Could you check a few things on this model? Use its own coordinates, in mm. A direction names the side the tool comes from. Give positions to 0.01 mm unless a question says otherwise; leave off trailing zeros. Loops run counter-clockwise (first coordinate to the right, second up) from the corner with the lowest first, then second, coordinate; pieces in that order, holes last. Notation, with made-up numbers: (34.5, 43) -> (59.5, 43) arc R30 ccw to (59.5, 71) -> close; hole circle Ø6 at (-24, 33.25). An arc over 180 degrees is marked (long way). Write each question's results on one line, items separated by ' | '. Start each with the question number.
Q1. We'd pull the mould along Y, two halves only. Please class faces 3 (the face through (-1, 1, 0)), 4 (the face through (-2.92, 7.56, 6.65)), 5 (the face through (-16.01, -72.08, 3.45)): released by +Y, released by -Y, zero draft, split by the parting line, or undercut.
Q2. If I drill on line 1 along Y through (x, z) = (0, 6.8); line 2 along Z through (x, y) = (-40.5, 53.5); line 3 along Y through (x, z) = (-28, 5.5), over which ranges is the centre line in solid material (lowest first)?
Q3. If we section it at C-C, the plane y = 55: List the corners of the cut face in (x, z) for me (3 decimals), plus the area to 3 significant figures.
Q4. If we section it at D-D, the plane x = 25: List the corners of the cut face in (y, z) for me.
Q5. If we section it at B-B, the plane z = 3.5: List the corners of the cut face in (x, y) for me, plus the area to 3 significant figures.
Q6. If we section it at A-A, the plane x = -44.5: List the corners of the cut face in (y, z) for me, plus the area to 3 significant figures.
Q7. Will these pins go through, and if not, where does the flat tip stop? P1, Ø0.8, axis at x = -8, z = 6.5, coming from the +Y side; P2, Ø4, axis at y = 24.5, z = 5.5, coming from the +X side; P3, Ø8, axis at x = -18.5, y = -49.5, coming from the -Z side; P4, Ø0.8, axis at x = -5, z = 6.5, coming from the +Y side.
Q8. Which directions (+Z, -Z, +X, -X, +Y, -Y) give clear straight access to the entire face, cutting with the end or side of a thin tool? Please do faces 1 (the face through (-6, -11, 7)), 2 (the face through (25.47, -19.885, 6.645)).
from build123d import *

# Parameters (mm, degrees)
F0_R     = 73.835319
F1_DEPTH = 7
F2_DEPTH = 6.3


with BuildPart() as f1:
    # F0 (on Top) → F1 (new body)
    with BuildSketch(Plane.XY):
        Circle(F0_R)
        with BuildLine():
            ThreePointArc((-55.352281, -38.118447), (-19.959771, 64.175529), (67.20782, 0))
            ThreePointArc((67.20782, 0), (29.467148, -60.403462), (-41.368183, -52.967579))
            ThreePointArc((-41.368183, -52.967579), (-48.926845, -46.076619), (-55.352281, -38.118447))
        make_face(mode=Mode.SUBTRACT)
        with BuildLine():
            Line((-50.618433, -35.51409), (-55.352281, -38.118447))
            ThreePointArc((-55.352281, -38.118447), (-48.926845, -46.076619), (-41.368183, -52.967579))
            Line((-41.368183, -52.967579), (-39.555106, -51.21921))
            Line((-39.555106, -51.21921), (-37.567016, -52.8697))
            Line((-37.567016, -52.8697), (-13.603393, -31.458031))
            Line((-13.603393, -31.458031), (1.234484, -14.347686))
            Line((1.234484, -14.347686), (1.234484, -12.075218))
            Line((1.234484, -12.075218), (11.05952, -6.03984))
            Line((11.05952, -6.03984), (32.11331, -34.933571))
            Line((32.11331, -34.933571), (34.920476, -38.40911))
            Line((34.920476, -38.40911), (37.861317, -40.547904))
            Line((37.861317, -40.547904), (46.550162, -43.221395))
            Line((46.550162, -43.221395), (46.899657, -42.085539))
            Line((46.899657, -42.085539), (37.076384, -35.29954))
            Line((37.076384, -35.29954), (13.533317, -4.032719))
            Line((13.533317, -4.032719), (16.463503, 0))
            Line((16.463503, 0), (13.533317, 2.129083))
            Line((13.533317, 2.129083), (13.533317, 5.39033))
            Line((13.533317, 5.39033), (11.05952, 5.39033))
            Line((11.05952, 5.39033), (11.05952, 8.130658))
            Line((11.05952, 8.130658), (9.254914, 8.130658))
            Line((9.254914, 8.130658), (9.188076, 9.868428))
            Line((9.188076, 9.868428), (4.174984, 9.675617))
            Line((4.174984, 9.675617), (-26.369359, 50.371822))
            Line((-26.369359, 50.371822), (-29.577548, 51.374383))
            Line((-29.577548, 51.374383), (-32.652061, 51.374383))
            Line((-32.652061, 51.374383), (-34.924529, 50.371822))
            Line((-34.924529, 50.371822), (-38.667418, 46.896283))
            Line((-38.667418, 46.896283), (-40.739372, 43.287069))
            Line((-40.739372, 43.287069), (-41.34091, 39.477345))
            Line((-41.34091, 39.477345), (-41.34091, 30.587986))
            Line((-41.34091, 30.587986), (-39.870489, 32.593105))
            Line((-39.870489, 32.593105), (-39.068446, 36.536504))
            Line((-39.068446, 36.536504), (-37.397511, 41.549303))
            Line((-37.397511, 41.549303), (-34.924529, 45.826886))
            Line((-34.924529, 45.826886), (-32.184202, 47.69833))
            Line((-32.184202, 47.69833), (-29.77806, 47.69833))
            Line((-29.77806, 47.69833), (-27.10457, 45.626376))
            Line((-27.10457, 45.626376), (-1.038028, 9.675617))
            Line((-1.038028, 9.675617), (-4.847753, 5.39033))
            Line((-4.847753, 5.39033), (-4.847753, 1.847953))
            Line((-4.847753, 1.847953), (-5.6498, 1.847953))
            Line((-5.6498, 1.847953), (-5.6498, -0.491352))
            Line((-5.6498, -0.491352), (-7.488666, -1.871504))
            Line((-7.488666, -1.871504), (-8.85799, -1.871504))
            Line((-8.85799, -1.871504), (-14.18264, -5.867895))
            Line((-14.18264, -5.867895), (-14.18264, -7.041406))
            Line((-14.18264, -7.041406), (-34.189317, -18.804768))
            Line((-34.189317, -18.804768), (-42.610817, -26.491057))
            Line((-42.610817, -26.491057), (-50.618433, -32.501136))
            Line((-50.618433, -32.501136), (-50.618433, -35.51409))
        make_face()
    extrude(amount=F1_DEPTH)

    # F0 (on Top) → F2 (join)
    with BuildSketch(Plane.XY):
        with BuildLine():
            ThreePointArc((-41.368183, -52.967579), (29.467148, -60.403462), (67.20782, 0))
            ThreePointArc((67.20782, 0), (-19.959771, 64.175529), (-55.352281, -38.118447))
            Line((-55.352281, -38.118447), (-50.618433, -35.51409))
            Line((-50.618433, -35.51409), (-50.618433, -32.501136))
            Line((-50.618433, -32.501136), (-42.610817, -26.491057))
            Line((-42.610817, -26.491057), (-34.189317, -18.804768))
            Line((-34.189317, -18.804768), (-14.18264, -7.041406))
            Line((-14.18264, -7.041406), (-14.18264, -5.867895))
            Line((-14.18264, -5.867895), (-8.85799, -1.871504))
            Line((-8.85799, -1.871504), (-7.488666, -1.871504))
            Line((-7.488666, -1.871504), (-5.6498, -0.491352))
            Line((-5.6498, -0.491352), (-5.6498, 1.847953))
            Line((-5.6498, 1.847953), (-4.847753, 1.847953))
            Line((-4.847753, 1.847953), (-4.847753, 5.39033))
            Line((-4.847753, 5.39033), (-1.038028, 9.675617))
            Line((-1.038028, 9.675617), (-27.10457, 45.626376))
            Line((-27.10457, 45.626376), (-29.77806, 47.69833))
            Line((-29.77806, 47.69833), (-32.184202, 47.69833))
            Line((-32.184202, 47.69833), (-34.924529, 45.826886))
            Line((-34.924529, 45.826886), (-37.397511, 41.549303))
            Line((-37.397511, 41.549303), (-39.068446, 36.536504))
            Line((-39.068446, 36.536504), (-39.870489, 32.593105))
            Line((-39.870489, 32.593105), (-41.34091, 30.587986))
            Line((-41.34091, 30.587986), (-41.34091, 39.477345))
            Line((-41.34091, 39.477345), (-40.739372, 43.287069))
            Line((-40.739372, 43.287069), (-38.667418, 46.896283))
            Line((-38.667418, 46.896283), (-34.924529, 50.371822))
            Line((-34.924529, 50.371822), (-32.652061, 51.374383))
            Line((-32.652061, 51.374383), (-29.577548, 51.374383))
            Line((-29.577548, 51.374383), (-26.369359, 50.371822))
            Line((-26.369359, 50.371822), (4.174984, 9.675617))
            Line((4.174984, 9.675617), (9.188076, 9.868428))
            Line((9.188076, 9.868428), (9.254914, 8.130658))
            Line((9.254914, 8.130658), (11.05952, 8.130658))
            Line((11.05952, 8.130658), (11.05952, 5.39033))
            Line((11.05952, 5.39033), (13.533317, 5.39033))
            Line((13.533317, 5.39033), (13.533317, 2.129083))
            Line((13.533317, 2.129083), (16.463503, 0))
            Line((16.463503, 0), (13.533317, -4.032719))
            Line((13.533317, -4.032719), (37.076384, -35.29954))
            Line((37.076384, -35.29954), (46.899657, -42.085539))
            Line((46.899657, -42.085539), (46.550162, -43.221395))
            Line((46.550162, -43.221395), (37.861317, -40.547904))
            Line((37.861317, -40.547904), (34.920476, -38.40911))
            Line((34.920476, -38.40911), (32.11331, -34.933571))
            Line((32.11331, -34.933571), (11.05952, -6.03984))
            Line((11.05952, -6.03984), (1.234484, -12.075218))
            Line((1.234484, -12.075218), (1.234484, -14.347686))
            Line((1.234484, -14.347686), (-13.603393, -31.458031))
            Line((-13.603393, -31.458031), (-37.567016, -52.8697))
            Line((-37.567016, -52.8697), (-39.555106, -51.21921))
            Line((-39.555106, -51.21921), (-41.368183, -52.967579))
        make_face()
    extrude(amount=F2_DEPTH)


solid = f1.part
Final values:
1) face 3: zero draft | face 4: undercut | face 5: split by the parting line
2) line 1: y = -73.84 to -67.21, -15.77 to 15.24, 67.21 to 73.84 | line 2: z = 0 to 6.3 | line 3: y = -68.32 to 68.32
3) outline: (-49.261, 0) -> (49.261, 0) -> (49.261, 7) -> (38.625, 7) -> (38.625, 6.3) -> (-38.625, 6.3) -> (-38.625, 7) -> (-49.261, 7) -> close | area: 636 mm²
4) outline: (-69.47, 0) -> (69.47, 0) -> (69.47, 7) -> (62.39, 7) -> (62.39, 6.3) -> (-19.26, 6.3) -> (-19.26, 7) -> (-25.17, 7) -> (-25.17, 6.3) -> (-62.39, 6.3) -> (-62.39, 7) -> (-69.47, 7) -> close
5) outline: circle Ø147.67 at (0, 0) | area: 17,100 mm²
6) outline: (-58.92, 0) -> (58.92, 0) -> (58.92, 7) -> (50.37, 7) -> (50.37, 6.3) -> (-27.91, 6.3) -> (-27.91, 7) -> (-58.92, 7) -> close | area: 770 mm²
7) P1: stops at y = 73.44 | P2: stops at x = 70.32 | P3: stops at z = 0 | P4: stops at y = 73.69
8) face 1: +Z, +X, -X, +Y, -Y | face 2: +Z
